```python
from build123d import *

# Parameters (mm, degrees)
SKETCH_1_W               = 90
SKETCH_1_H               = 35
EXTRUDE_1_DEPTH          = 3
SKETCH_2_W               = 5
SKETCH_2_H               = 6
EXTRUDE_2_DEPTH          = 5
SKETCH_3_R               = 1.25
CUT_EXTRUDE_1_DEPTH      = 97.896852374
SKETCH_4_W               = 6
SKETCH_4_H               = 6
EXTRUDE_3_DEPTH          = 6
CUT_EXTRUDE_2_DEPTH      = 95.25099469
CUT_EXTRUDE_2_DEPTH_BACK = 95.25099469
SKETCH_5_R               = 1.25


with BuildPart() as part:
    # Эскиз1 → Бобышка-Вытянуть1 (new body)
    with BuildSketch(Plane(origin=(0, 0, 0), x_dir=(0, 0, -1), z_dir=(1, 0, 0))):
        with Locations((45, 17.5)):
            Rectangle(SKETCH_1_W, SKETCH_1_H)
    extrude(amount=EXTRUDE_1_DEPTH)

    # Эскиз2 → Бобышка-Вытянуть2 (add)
    with BuildSketch(Plane(origin=(3, 0, 0), x_dir=(0, 0, -1), z_dir=(1, 0, 0))):
        with Locations((2.5, 32)):
            Rectangle(SKETCH_2_W, SKETCH_2_H)
        with Locations((2.5, 3)):
            Rectangle(SKETCH_2_W, SKETCH_2_H)
    extrude(amount=EXTRUDE_2_DEPTH)

    # Эскиз3 → Вырез-Вытянуть1 (cut, through all)
    with BuildSketch(Plane(origin=(0, 0, 0), x_dir=(-1, 0, 0), z_dir=(0, -1, 0))):
        with Locations(Location((-5.5, 2.5, 0), (0, 0, 90))):
            Circle(SKETCH_3_R)
        with BuildLine():
            Line((-8, 5), (-8, 2.5))
            ThreePointArc((-8, 2.5), (-7.267766953, 4.267766953), (-5.5, 5))
            Line((-5.5, 5), (-8, 5))
        make_face()
        with BuildLine():
            Line((-8, 0), (-5.5, 0))
            ThreePointArc((-5.5, 0), (-7.267766953, 0.732233047), (-8, 2.5))
            Line((-8, 2.5), (-8, 0))
        make_face()
    extrude(amount=-CUT_EXTRUDE_1_DEPTH, mode=Mode.SUBTRACT)

    # Эскиз4 → Бобышка-Вытянуть3 (add)
    with BuildSketch(Plane(origin=(3, 0, 0), x_dir=(0, 0, -1), z_dir=(1, 0, 0))):
        with Locations((57, 23.5)):
            Rectangle(SKETCH_4_W, SKETCH_4_H)
        with Locations((57, 11.5)):
            Rectangle(SKETCH_4_W, SKETCH_4_H)
    extrude(amount=EXTRUDE_3_DEPTH)

    # Эскиз5 → Вырез-Вытянуть2 (cut, two sides: drawn at the far end of the back side and taken through both)
    with BuildSketch(Plane(origin=(0, 8.5, 0), x_dir=(-1, 0, 0), z_dir=(0, -1, 0)).offset(-CUT_EXTRUDE_2_DEPTH_BACK)):
        with Locations(Location((-6, 57, 0), (0, 0, 90))):
            Circle(SKETCH_5_R)
        with BuildLine():
            Line((-9, 60), (-9, 57.000000015))
            ThreePointArc((-9, 57.000000015), (-8.121320338, 59.121320349), (-6, 60))
            Line((-6, 60), (-9, 60))
        make_face()
        with BuildLine():
            Line((-9, 54), (-6, 54))
            ThreePointArc((-6, 54), (-8.121320349, 54.878679662), (-9, 57.000000015))
            Line((-9, 57.000000015), (-9, 54))
        make_face()
    extrude(amount=CUT_EXTRUDE_2_DEPTH + CUT_EXTRUDE_2_DEPTH_BACK, mode=Mode.SUBTRACT)


solid = part.part
```
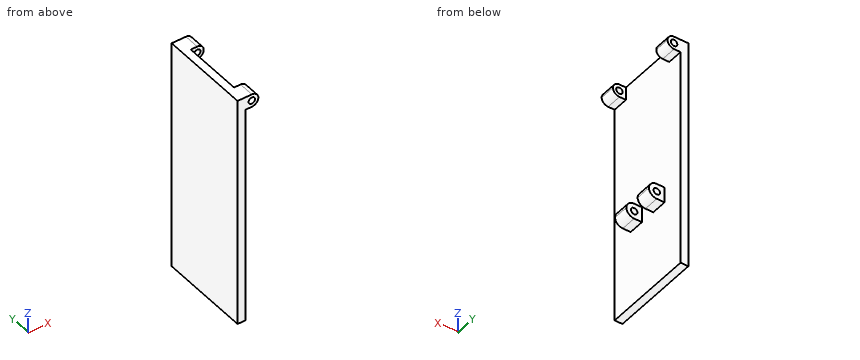
Geometry check sheet. Reference: the model listing, model coordinates, mm. Round coordinates to 2 decimals unless told otherwise and drop trailing zeros. Order: outer loops, then holes, each group sorted by start corner. A loop starts at its lowest first (then second) coordinate and runs counter-clockwise, first axis right, second up. Notation, with made-up numbers: (53.25, 48.25) - (82.25, 48.25) arc R29 ccw to (82.25, 86.25) - close; hole circle Ø11 at (6, 72). An arc over 180 degrees is marked (long way). Use a Markdown table: item, result. Add a question column.
(1) Sectioned sample at A-A, the plane y = 31.5. Enter the section's corners in (x, z).
(2) Sectioned sample at B-B, the plane z = -46. Enter the section's corners in (x, y), and give its area (3 significant figures).
(3) Depth check by flat-ended pin: pin 1 (3.5 mm diameter, centred on x = 5, y = 13, fed in from +Z); pin 2 (4 mm diameter, centred on y = 17, z = -25, fed in from -X); pin 3 (3.5 mm diameter, centred on x = 5, y = 25, fed in from -Z); pin 4 (1.2 mm diameter, centred on x = 4.5, y = 3.5, fed in from -Z). Enter the tip coordinate at first touch or a pass-through.
(4) Material ranges on line 1 along X through (y, z) = (13, -57); line 2 along Z through (x, y) = (6, 10.5); line 3 along Y through (x, z) = (6.5, -4.5), recorded low to high. Write a range as [from, to].
Answers below:
| question | item | result |
|---|---|---|
| 1 | outline | (0, -90) - (3, -90) - (3, -5) - (5.5, -5) arc R2.5 ccw to (5.5, 0) - (0, 0) - close; hole circle Ø2.5 at (5.5, -2.5) |
| 2 | outline | (0, 0) - (3, 0) - (3, 35) - (0, 35) - close |
| 2 | area | 105 mm² |
| 3 | pin 1 | z = -54 |
| 3 | pin 2 | x = 0 |
| 3 | pin 3 | z = -60 |
| 3 | pin 4 | z = -5 |
| 4 | line 1 | [0, 4.75], [7.25, 9] |
| 4 | line 2 | [-60, -58.25], [-55.75, -54] |
| 4 | line 3 | [0, 6], [29, 35] |
